Model file for the job. Use its own axes, mm. Face numbers are marked on the shaded views. A direction names the side the tool comes from. Round coordinates to 2 decimals unless told otherwise and drop trailing zeros. Order: outer loops, then holes, each group sorted by start corner. A loop starts at its lowest first (then second) coordinate and runs counter-clockwise, first axis right, second up. Notation, with made-up numbers: (30, 62.5) - (63, 62.5) arc R6 ccw to (63, 73.5) - close; hole circle Ø6 at (-27, -20.5). An arc over 180 degrees is marked (long way). Put each result on its own line as item: value. Start each with the question number.
Item 1: Pin check, flat tips, straight feed: pin 1 Ø12 at (x, y) = (1148.5, 116) entering from +Z; pin 2 Ø10 at (x, y) = (1027, 77.5) entering from -Z; pin 3 Ø3 at (x, y) = (1033, -66) entering from -Z. Stop position of each tip, or through.
Item 2: Saw through at C-C on x = 1129.5. List the corners of the cut face in (y, z).
Item 3: Mould opens along Z. For the marked faces 3, 4 and 5 say: pulls with the +Z half, pulls with the -Z half, needs draft (parallel to the pull), parting line crosses it, or undercut.
Item 4: Which spindle directions (+Z, -Z, +X, -X, +Y, -Y) get a long thin tool onto all of the face, cutting with end or side? Do the marked faces 1 and 2. Say none if no direction does.
Item 5: Saw through at A-A on y = 0. List the corners of the cut face in (x, z), plus the area to 4 significant figures.
Item 6: Probe probe 1 along X at (y, z) = (-23.5, -142.5); probe 2 along Z at (x, y) = (1130.5, 130); probe 3 along Y at (x, z) = (1153, -6). List the from-to ranges inside material, lowest first.
Item 7: Saw through at D-D on x = 1035. List the corners of the cut face in (y, z).
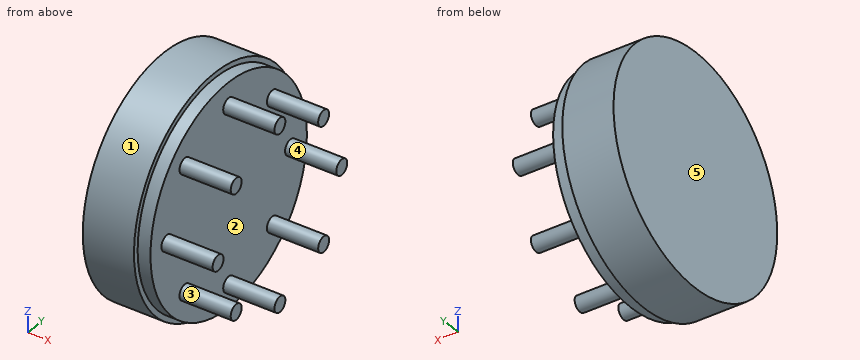
```python
from build123d import *

# Parameters (mm, degrees)
SKETCH2_R           = 215
BOSS_EXTRUDE1_DEPTH = 25
SKETCH3_R           = 225
BOSS_EXTRUDE2_DEPTH = 100
SKETCH5_R           = 15
BOSS_EXTRUDE3_DEPTH = 100


with BuildPart() as part:
    # Sketch2 → Boss-Extrude1 (new body)
    with BuildSketch(Plane(origin=(1124.08, 0, 0), x_dir=(0, 0, -1), z_dir=(1, 0, 0))):
        Circle(SKETCH2_R)
    extrude(amount=-BOSS_EXTRUDE1_DEPTH)

    # Sketch3 → Boss-Extrude2 (add)
    with BuildSketch(Plane.ZY.offset(-1099.08)):
        Circle(SKETCH3_R)
    extrude(amount=BOSS_EXTRUDE2_DEPTH)

    # Sketch5 → Boss-Extrude3 (add)
    with BuildSketch(Plane(origin=(1124.08, 0, 0), x_dir=(0, 0, -1), z_dir=(1, 0, 0))):
        with Locations((0, 170)):
            Circle(SKETCH5_R)
        with Locations((120.208152802, 120.208152802)):
            Circle(SKETCH5_R)
        with Locations((170, 0)):
            Circle(SKETCH5_R)
        with Locations((120.208152802, -120.208152802)):
            Circle(SKETCH5_R)
        with Locations((0, -170)):
            Circle(SKETCH5_R)
        with Locations((-120.208152802, -120.208152802)):
            Circle(SKETCH5_R)
        with Locations((-170, 0)):
            Circle(SKETCH5_R)
        with Locations((-120.208152802, 120.208152802)):
            Circle(SKETCH5_R)
    extrude(amount=BOSS_EXTRUDE3_DEPTH)


solid = part.part
```
Results found:
1. pin 1: stops at z = 135.21
1. pin 2: stops at z = -213
1. pin 3: stops at z = -215.56
2. outline: circle Ø30 at (-170, 0); circle Ø30 at (-120.21, -120.21); circle Ø30 at (-120.21, 120.21); circle Ø30 at (0, -170); circle Ø30 at (0, 170); circle Ø30 at (120.21, -120.21); circle Ø30 at (120.21, 120.21); circle Ø30 at (170, 0)
3. face 3: undercut
3. face 4: parting line crosses it
3. face 5: needs draft
4. face 1: +X, -X
4. face 2: +X
5. outline: (999.08, -225) - (1099.08, -225) - (1099.08, -215) - (1124.08, -215) - (1124.08, -185) - (1224.08, -185) - (1224.08, -155) - (1124.08, -155) - (1124.08, 155) - (1224.08, 155) - (1224.08, 185) - (1124.08, 185) - (1124.08, 215) - (1099.08, 215) - (1099.08, 225) - (999.08, 225) - close
5. area: 61,750 mm²
6. probe 1: x = 999.08 to 1124.08
6. probe 2: z = -131.57 to -108.85, 108.85 to 131.57
6. probe 3: y = -183.75 to -156.25, 156.25 to 183.75
7. outline: circle Ø450 at (0, 0)
